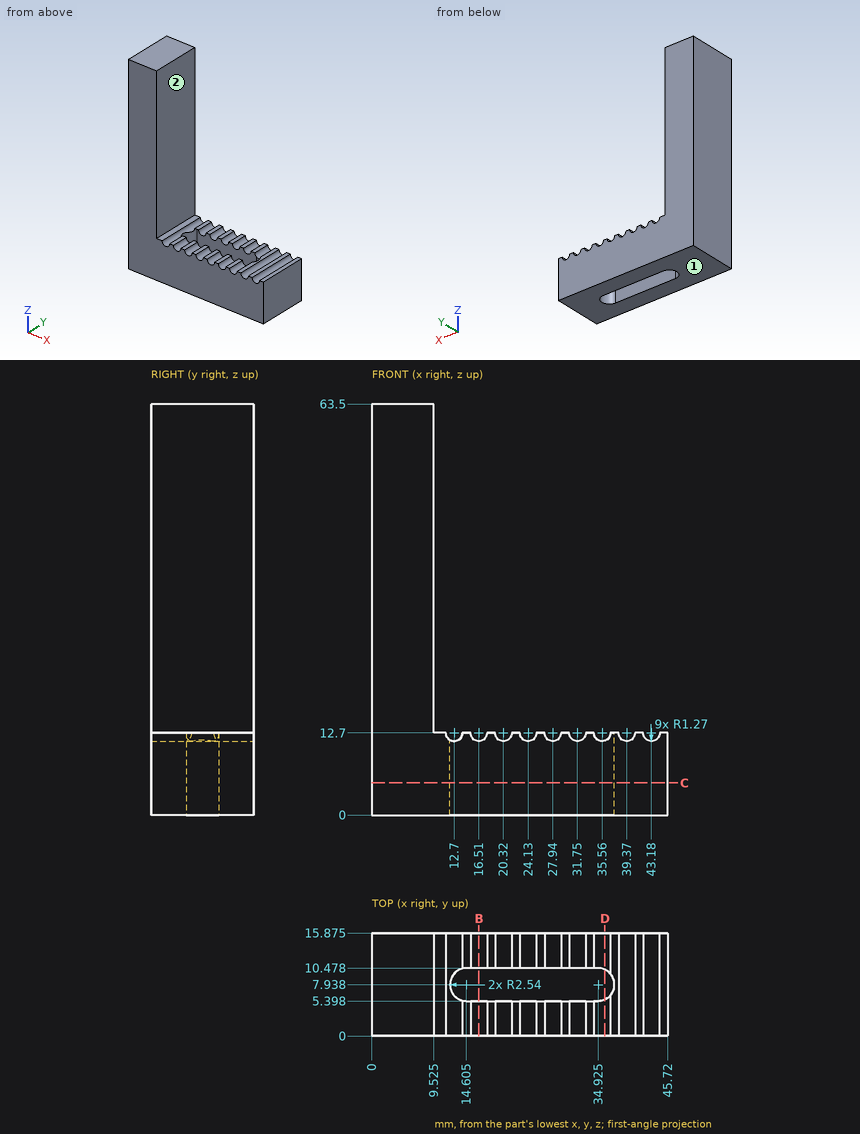
Answer from the drawing. Dimensions are ordinates in mm from the lowest x, y and z of the part. A direction names the side the tool comes from. Round coordinates to 2 decimals unless told otherwise and drop trailing zeros. Loops run counter-clockwise (first coordinate to the right, second up) from the corner with the lowest first, then second, coordinate; pieces in that order, holes last. Notation, with made-up numbers: (-12.75, 44) - (35.25, 44) arc R15 cw to (35.25, 56) - close; hole circle Ø3 at (45, 56). An arc over 180 degrees is marked (long way). Return JSON: item names as keys, results as strings. Group by question number.
1. The part is cut by section D-D on x = 36. Determine the outline of the cut face in (y, z) (1 decimal), then the cut area to 3 significant figures.
2. The part is cut by section C-C on z = 5. Determine the outline of the cut face in (x, y) (1 decimal), then the cut area to 3 significant figures.
3. Which of the six approach directions +Z, -Z, +X, -X, +Y, -Y give full straight-line access (tool end or side, diameter ignored) to the marked faces 1 and 2?
4. Each of these flat-tipped pins is pushed along its axis until it touches: P1, Ø1.4, axis at x = 37.5, y = 9.5, coming from the +Z side; P2, Ø2, axis at y = 14, z = 38.5, coming from the +X side (1 decimal). Where does it stop, or does it pass through?
5. The part is cut by section B-B on x = 16.51. Determine the outline of the cut face in (y, z) (1 decimal), then the cut area to 3 significant figures.
6. Consider probe 1 along Y at (x, z) = (35, 8) (1 decimal); probe 2 along X at (y, z) = (5.25, 50.5) (1 decimal); probe 3 along Z at (x, y) = (22, 5). Determine where each line is inside the solid, lowest interval first.
Resolved:
{
 "1": {"outline": "(0, 0) - (5.6, 0) - (5.6, 11.5) - (0, 11.5) - close; (10.2, 0) - (15.9, 0) - (15.9, 11.5) - (10.2, 11.5) - close", "area": "130 mm²"},
 "2": {"outline": "(0, 0) - (45.7, 0) - (45.7, 15.9) - (0, 15.9) - close; hole (14.6, 5.4) - (34.9, 5.4) arc R2.5 ccw to (34.9, 10.5) - (14.6, 10.5) arc R2.5 ccw to start", "area": "602 mm²"},
 "3": {"face 1": "-Z, +X, -X, +Y, -Y", "face 2": "+Z, +X, +Y, -Y"},
 "4": {"P1": "stops at z = 12.7", "P2": "stops at x = 9.5"},
 "5": {"outline": "(0, 0) - (5.4, 0) - (5.4, 11.4) - (0, 11.4) - close; (10.5, 0) - (15.9, 0) - (15.9, 11.4) - (10.5, 11.4) - close", "area": "123 mm²"},
 "6": {"probe 1": "y = 0 to 5.4, 10.5 to 15.9", "probe 2": "x = 0 to 9.5", "probe 3": "z = 0 to 12.7"}
}
